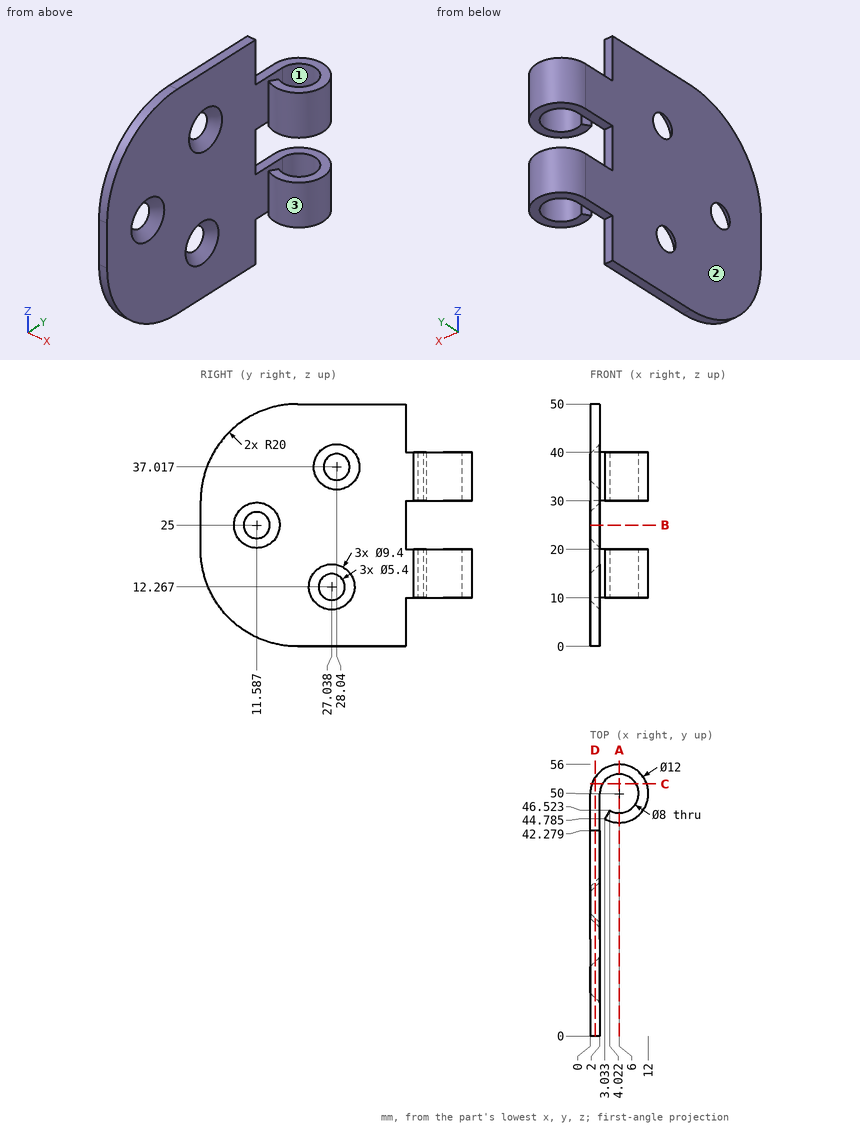
Print and shaded views of the part. All mm, measured from the part's lowest x, y and z. Give positions to 0.01 mm unless a question says otherwise; leave off trailing zeros. Order: outer loops, then holes, each group sorted by start corner. A loop starts at its lowest first (then second) coordinate and runs counter-clockwise, first axis right, second up. Notation, with made-up numbers: (-10, 37) -> (6, 37) arc R11 cw to (6, 53) -> close; hole circle Ø1 at (-32, -18.75). An arc over 180 degrees is marked (long way). Use CSV: the item, a comma, the result in double quotes.
1. Band-saw the part on C-C, the plane y = 52. Give the cut face in (x, z) (1 decimal).
Outcome:
outline,"(0.3, 10) -> (2.5, 10) -> (2.5, 20) -> (0.3, 20) -> close; (0.3, 30) -> (2.5, 30) -> (2.5, 40) -> (0.3, 40) -> close; (9.5, 10) -> (11.7, 10) -> (11.7, 20) -> (9.5, 20) -> close; (9.5, 30) -> (11.7, 30) -> (11.7, 40) -> (9.5, 40) -> close"
2. Mould opens along Y. For the marked faces 1, 2 and 3 say: +Y half, -Y half, draft (parallel to the pull), parting line (faces both ways), or undercut.
Outcome:
face 1,"undercut"
face 2,"draft"
face 3,"parting line"
3. Band-saw the part on A-A, the plane x = 6. Give the cut face in (y, z).
Outcome:
outline,"(44, 10) -> (46, 10) -> (46, 20) -> (44, 20) -> close; (44, 30) -> (46, 30) -> (46, 40) -> (44, 40) -> close; (54, 10) -> (56, 10) -> (56, 20) -> (54, 20) -> close; (54, 30) -> (56, 30) -> (56, 40) -> (54, 40) -> close"
4. Drop flat-ended pins along their axis: pin 1 (4 mm diameter, centred on x = 3, z = 42.5, fed in from +Y); pin 2 (4 mm diameter, centred on y = 48, z = 41.5, fed in from +X); pin 3 (7 mm diameter, centred on x = 6, y = 50, fed in from +Z); pin 4 (4 mm diameter, centred on y = 16, z = 25, fed in from +X). Give the stop position or say it passes through.
Outcome:
pin 1,"y = 42.28"
pin 2,"x = 11.96"
pin 3,"through"
pin 4,"x = 2"
5. Band-saw the part on B-B, the plane z = 25. Give the cut face in (x, y).
Outcome:
outline,"(0, 0) -> (2, 0) -> (2, 6.89) -> (0, 8.89) -> close; (0, 14.29) -> (2, 16.29) -> (2, 42.28) -> (0, 42.28) -> close"
6. Drill centre lines: line 1 along Y through (x, z) = (6, 32); line 2 along X through (y, z) = (38.5, 43); line 3 along X through (y, z) = (50, 16). Where is each one in solid material? Low to high. Write a range as from..to.
Outcome:
line 1,"44..46, 54..56"
line 2,"0..2"
line 3,"0..2, 10..12"
7. Band-saw the part on D-D, the plane x = 1. Give the cut face in (y, z), then the cut area to 3 significant figures.
Outcome:
outline,"(0, 20) arc R20 ccw to (20, 0) -> (42.28, 0) -> (42.28, 10) -> (53.32, 10) -> (53.32, 20) -> (42.28, 20) -> (42.28, 30) -> (53.32, 30) -> (53.32, 40) -> (42.28, 40) -> (42.28, 50) -> (20, 50) arc R20 ccw to (0, 30) -> close; hole circle Ø7.4 at (11.59, 25); hole circle Ø7.4 at (27.04, 12.27); hole circle Ø7.4 at (28.04, 37.02)"
area,"2,030 mm²"
